Check sheet for the modelled part. Datum: model origin and axes. Units: mm. A direction names the side the tool comes from. Round coordinates to 2 decimals unless told otherwise and drop trailing zeros. Write each loop counter-clockwise with the first axis right and the second up, starting at its lowest first coordinate (ties: lowest second). Pieces come first, ordered by that corner, then holes. Notation, with made-up numbers: (35.5, 57.5) -> (69.5, 57.5) arc R19 ccw to (69.5, 91.5) -> close; hole circle Ø3 at (-6.75, 21). An arc over 180 degrees is marked (long way). One line per item, written item: value. Start each with the question number.
Autodesk Inventor part; units mm, degrees
ref_plane "YZ Plane" through (0, 0, 0) normal (1, 0, 0) x (0, 1, 0)
ref_plane "XZ Plane" through (0, 0, 0) normal (0, 1, 0) x (-1, 0, 0)
ref_plane "XY Plane" through (0, 0, 0) normal (0, 0, 1) x (1, 0, 0)
sketch "Sketch1" plane through (0, 0, 0) normal (0, 0, 1) x (1, 0, 0)
  line L0 (0, 0) -> (0, 719.074)
  line L1 (0, 719.074) -> (342.9, 719.074)
  line L2 (0, 0) -> (342.9, 0)
  line L3 (342.9, 801.624) -> (-82.55, 801.624)
  line L4 (-82.55, 801.624) -> (-82.55, -82.55)
  line L5 (-82.55, -82.55) -> (342.9, -82.55)
  line L6 (342.9, 719.074) -> (342.9, 801.624)
  line L7 (342.9, 0) -> (342.9, -82.55)
  dimension "d0" = 719.074
  dimension "d1" = 342.9
  dimension "d2" = 82.55
extrude "Extrusion1" add sketch "Sketch1" along normal blind 127
fillet "Fillet1" radius 25.4 8 edges at (130.175, 801.624, 127) (130.175, 801.624, 0) (-82.55, 801.624, 63.5) (-82.55, 359.537, 127) (-82.55, 359.537, 0) (-82.55, -82.55, 63.5) (130.175, -82.55, 0) (130.175, -82.55, 127)
sketch "Sketch2" plane through (0, 719.074, 0) normal (0, -1, 0) x (1, 0, 0)
  line L0 (342.9, 0) -> (342.9, 127) construction
  line L1 (0, 127) -> (342.9, 127) construction
  line L2 (0, 127) -> (190.5, 127) construction
  line L3 (0, 0) -> (342.9, 0) construction
  line L4 (190.5, 0) -> (190.5, 97.282) construction
  line L5 (190.5, 0) -> (287.782, 0) construction
  line L6 (190.5, 97.282) -> (215.9, 97.282) construction
  circle A0 centre (190.5, 97.282) radius 2.5797
  circle A1 centre (215.9, 97.282) radius 2.5797
  dimension "d30" = 190.5
  dimension "d31" = 97.282
  dimension "d32" = 90
  dimension "d33" = 25.4
  dimension "d34" = 5.1594
sketch "Sketch3" plane through (0, 0, 0) normal (0, 1, 0) x (1, 0, 0)
  line L0 (0, 0) -> (0, -127) construction
  line L1 (0, -127) -> (190.5, -127) construction
  line L2 (342.9, -127) -> (0, -127) construction
  line L3 (190.5, -127) -> (190.5, -97.282) construction
  line L4 (190.5, -127) -> (220.218, -127) construction
  line L5 (190.5, -97.282) -> (215.9, -97.282) construction
  line L6 (190.5, -97.282) -> (215.9, -97.282) construction
  circle A0 centre (190.5, -97.282) radius 2.5797
  circle A1 centre (215.9, -97.282) radius 2.5797
  dimension "d37" = 190.5
  dimension "d38" = 29.718
  dimension "d39" = 90
  dimension "d40" = 25.4
  dimension "d41" = 0
  dimension "d42" = 5.1594
sketch "Sketch4" plane through (0, 0, 0) normal (1, 0, 0) x (0, 0, -1)
  line L0 (-127, -57.15) -> (-127, 0) construction
  line L1 (-127, 0) -> (-127, 207.137) construction
  line L2 (-127, 0) -> (-127, 719.074) construction
  line L3 (-127, 207.137) -> (-55.118, 207.137) construction
  line L4 (-55.118, 207.137) -> (-36.068, 207.137) construction
  line L5 (-36.068, 207.137) -> (-17.018, 207.137) construction
  circle A0 centre (-55.118, 207.137) radius 2.667
  circle A1 centre (-36.068, 207.137) radius 2.667
  circle A2 centre (-17.018, 207.137) radius 2.667
  line L6 (-127, 359.537) -> (0, 359.537) construction
  line L7 (0, 0) -> (0, 719.074) construction
  line L8 (-55.118, 511.937) -> (-36.068, 511.937) construction
  line L9 (-36.068, 511.937) -> (-17.018, 511.937) construction
  circle A3 centre (-55.118, 511.937) radius 2.667
  circle A4 centre (-36.068, 511.937) radius 2.667
  circle A5 centre (-17.018, 511.937) radius 2.667
  dimension "d23" = 207.137
  dimension "d24" = 71.882
  dimension "d25" = 19.05
  dimension "d26" = 19.05
  dimension "d27" = 5.334
extrude "Extrusion4" cut sketch "Sketch4" against normal blind 4.7625
extrude "Extrusion5" cut sketch "Sketch2" against normal blind 25.4
extrude "Extrusion6" cut sketch "Sketch3" against normal blind 25.4
properties part number "Bumper Side V2"
1. Depth check by flat-ended pin: pin 1 Ø6 at (y, z) = (512, 16) entering from +X; pin 2 Ø6 at (y, z) = (511.937, 17.018) entering from -X; pin 3 Ø10 at (y, z) = (205, 107.5) entering from -X. Enter the tip coordinate at first touch or a pass-through.
2. Cross-section at B-B (z = 75.5). Record the cut outline in (x, y), plus the area to 3 significant figures.
3. Material ranges on probe 1 along Y at (x, z) = (205.5, 74); probe 2 along Z at (x, y) = (190, 738); probe 3 along X at (y, z) = (82.5, 83.5), recorded low to high.
4. Cross-section at A-A (x = 283.5). Record the cut outline in (y, z), plus the area to 3 significant figures.
5. Access from +Z, -Z, +X, -X, +Y, -Y to the whole of each face (thin tool, end or side, straight path). Record for faces 1 (the face through (169, 719.074, 63)), 2 (the face through (-82.55, 365, 63)).
6. Cross-section at C-C (y = 128). Record the cut outline in (x, z).
Working result:
1. pin 1: stops at x = 0
1. pin 2: stops at x = -81.97
1. pin 3: stops at x = -82.53
2. outline: (-82.55, -57.15) arc R25.4 ccw to (-57.15, -82.55) -> (342.9, -82.55) -> (342.9, 0) -> (0, 0) -> (0, 719.07) -> (342.9, 719.07) -> (342.9, 801.62) -> (-57.15, 801.62) arc R25.4 ccw to (-82.55, 776.22) -> close
2. area: 129,000 mm^2
3. probe 1: y = -82.55 to 0, 719.07 to 801.62
3. probe 2: z = 0 to 94.75, 99.81 to 127
3. probe 3: x = -82.55 to 0
4. outline: (-82.55, 25.4) arc R25.4 ccw to (-57.15, 0) -> (0, 0) -> (0, 127) -> (-57.15, 127) arc R25.4 ccw to (-82.55, 101.6) -> close; (719.07, 0) -> (776.22, 0) arc R25.4 ccw to (801.62, 25.4) -> (801.62, 101.6) arc R25.4 ccw to (776.22, 127) -> (719.07, 127) -> close
4. area: 20,400 mm^2
5. face 1: +Z, -Z, +X
5. face 2: +Z, -Z, -X, +Y, -Y
6. outline: (-82.55, 25.4) arc R25.4 ccw to (-57.15, 0) -> (0, 0) -> (0, 127) -> (-57.15, 127) arc R25.4 ccw to (-82.55, 101.6) -> close
